Solid Edge part; units mm, degrees
sketch "Sketch1" plane through (0, 0, 0) normal (0, 0, 1) x (1, 0, 0)
  line L0 (-165.1, -76.2) -> (165.1, -76.2)
  line L1 (165.1, -76.2) -> (165.1, 76.2)
  line L2 (165.1, 76.2) -> (-165.1, 76.2)
  line L3 (-165.1, 76.2) -> (-165.1, -76.2)
  dimension "D1" = 165.1
  dimension "D2" = 165.1
extrude "Protrusion1" add sketch "Sketch1" along normal blind 19.05
sketch "Sketch2" plane through (0, 0, 19.05) normal (0, 0, 1) x (1, 0, 0)
  line L0 (99.568, -6.35) -> (150.368, -6.35)
  line L1 (150.368, -6.35) -> (150.368, 6.35)
  line L2 (150.368, 6.35) -> (99.568, 6.35)
  line L3 (99.568, 6.35) -> (99.568, -6.35)
  dimension "D1" = 150.368
  dimension "D2" = 150.368
extrude "ExtrudedCutout_2" cut sketch "Sketch2" against normal blind 25.4
sketch "Sketch3" plane through (0, 0, 19.05) normal (0, 0, 1) x (0, -1, 0)
  circle A0 centre (-12.065, 107.188) radius 3.175
  circle A1 centre (-12.065, 142.748) radius 3.175
  dimension "D1" = 12.065
extrude "TopPivotMountHole12" cut sketch "Sketch3" against normal blind 25.4
mirror "Mirror1" about plane through (0, 0, 0) normal (0, -1, 0) of "TopPivotMountHole12"
properties material "Wood, Oak"
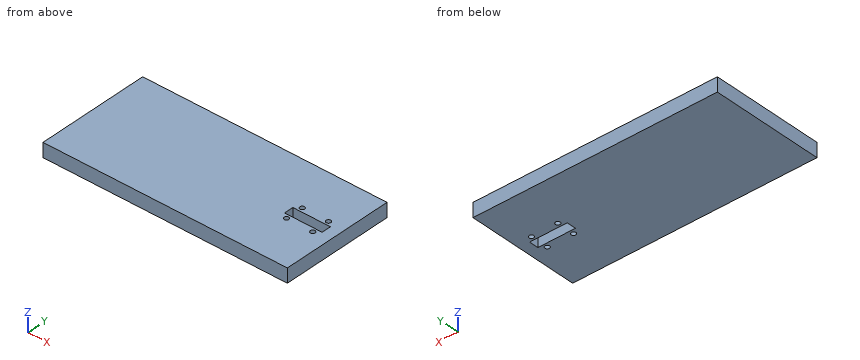
Verification items for the finished model (mm, model axes). Round coordinates to 2 decimals unless told otherwise and drop trailing zeros. Order: outer loops, then holes, each group sorted by start corner. A loop starts at its lowest first (then second) coordinate and runs counter-clockwise, first axis right, second up. Notation, with made-up numbers: (45.5, 66.5) - (102.5, 66.5) arc R28 ccw to (102.5, 97.5) - close; hole circle Ø3 at (45.25, -36). An arc over 180 degrees is marked (long way). Use CSV: the item, a comma, the result in double quotes.
(1) Section check A-A on x = 122. Record the boundary of the cut face in (y, z).
Entries:
outline,"(-76.2, 0) - (-6.35, 0) - (-6.35, 19.05) - (-76.2, 19.05) - close; (6.35, 0) - (76.2, 0) - (76.2, 19.05) - (6.35, 19.05) - close"
(2) Thickness scan on probe 1 along Y at (x, z) = (143, 2); probe 2 along Y at (x, z) = (136, 14.25); probe 3 along X at (y, z) = (-1, 11). Record the ranges inside material, lowest first. Write a range as from..to.
Entries:
probe 1,"-76.2..-15.23, -8.9..-6.35, 6.35..8.9, 15.23..76.2"
probe 2,"-76.2..-6.35, 6.35..76.2"
probe 3,"-165.1..99.57, 150.37..165.1"
(3) Section check B-B on z = 8.75. Record the boundary of the cut face in (x, y) (3 decimals), and give its area (3 significant figures).
Entries:
outline,"(-165.1, -76.2) - (165.1, -76.2) - (165.1, 76.2) - (-165.1, 76.2) - close; hole (99.568, -6.35) - (150.368, -6.35) - (150.368, 6.35) - (99.568, 6.35) - close; hole circle Ø6.35 at (107.188, -12.065); hole circle Ø6.35 at (107.188, 12.065); hole circle Ø6.35 at (142.748, -12.065); hole circle Ø6.35 at (142.748, 12.065)"
area,"49,600 mm^2"
(4) Gauge pin test, flat end, axial feed: pin 1 Ø6 at (x, y) = (-91, -10.5) entering from -Z. Record the tip position at first contact, or that the pin passes through.
Entries:
pin 1,"z = 0"
